from build123d import *

# Parameters (mm, degrees)
SKETCH_R           = 34
SKETCH_R_2         = 27
PAD_DEPTH          = 1.5
SKETCH001_W        = 1.2
SKETCH001_H        = 2
PAD001_DEPTH       = 0.1
SKETCH002_R        = 1
POCKET_DEPTH       = 1.601
SKETCH003_W        = 5
SKETCH003_H        = 5
PAD002_DEPTH       = 1.5
POLARPATTERN_COUNT = 16


with BuildPart() as part:
    # Sketch → Pad (new body)
    with BuildSketch(Plane.XY):
        Circle(SKETCH_R)
        Circle(SKETCH_R_2, mode=Mode.SUBTRACT)
    extrude(amount=PAD_DEPTH)

    # Sketch001 (on Face3 of Pad) → Pad001 (join)
    with BuildSketch(Plane(origin=(0, 0, 0), x_dir=(1, 0, 0), z_dir=(0, 0, -1))):
        with Locations((-3.4, 31.5)):
            Rectangle(SKETCH001_W, SKETCH001_H)
        with Locations((-1.133333, 31.5)):
            Rectangle(SKETCH001_W, SKETCH001_H)
        with Locations((1.133333, 31.5)):
            Rectangle(SKETCH001_W, SKETCH001_H)
        with Locations((3.4, 31.5)):
            Rectangle(SKETCH001_W, SKETCH001_H)
    extrude(amount=PAD001_DEPTH)

    # Sketch002 (on Face3 of Pad001) → Pocket (cut, through all)
    with BuildSketch(Plane.XY.offset(1.5)):
        with Locations((-26.5, 17.5)):
            Circle(SKETCH002_R)
        with Locations((26.5, 17.5)):
            Circle(SKETCH002_R)
        with Locations((26.5, -17.5)):
            Circle(SKETCH002_R)
        with Locations((-26.5, -17.5)):
            Circle(SKETCH002_R)
    extrude(amount=-POCKET_DEPTH, mode=Mode.SUBTRACT)

    # Sketch003 (on Face3 of Pocket) → Pad002 (join)
    with BuildSketch(Plane.XY.offset(1.5)):
        with Locations((0, 29.5)):
            Rectangle(SKETCH003_W, SKETCH003_H)
    pad002 = extrude(amount=PAD002_DEPTH)

    # PolarPattern: Pad002 ×16 about axis
    polarpattern_axis = Axis((0, 0, 1.5), (0, 0, 1))
    for i in range(1, POLARPATTERN_COUNT):
        add(pad002.rotate(polarpattern_axis, i * 360 / POLARPATTERN_COUNT))


solid = part.part
Work out the finished part from the listing and answer in its coordinate system (mm). A direction names the side the tool comes from. Give positions to 0.01 mm unless a question says otherwise; leave off trailing zeros. Loops run counter-clockwise (first coordinate to the right, second up) from the corner with the lowest first, then second, coordinate; pieces in that order, holes last. Notation, with made-up numbers: (31, 9.25) - (72, 9.25) arc R29 ccw to (72, 29.25) - close; hole circle Ø1 at (-23.75, 1.25). An arc over 180 degrees is marked (long way). Answer in a Markdown table with one row per item. Add a question column.
Q1. The part is cut by section B-B (y = 13.5). Determine the outline of the cut face in (x, z).
Q2. Consider line 1 along X through (y, z) = (-29, 2.75); line 2 along X through (y, z) = (1, 0.9); line 3 along Y through (x, z) = (-11, 0.15). Determine where each line is inside the solid, lowest interval first.
Q3. The part is cut by section C-C (x = -23). Determine the outline of the cut face in (y, z).
Q4. A tool of negligible diameter and unlimited length cuts with its end or side. For faces 1 (the flat face through (-22.603, -22.652, 2.24)), 2 (the flat face through (-10.365, 24.931, 2.24)), 3 (the flat face through (22.603, -19.067, 2.24)), 4 (the flat face through (2.5, 29, 2)), 5 (the flat face through (-8.966, -28.179, 2.24)), from which of +Z, -Z, +X, -X, +Y, -Y can it reach the whole face along a straight path? Write none if from no direction.
Q5. Each of these flat-tipped pins is pushed along its axis until it touches: P1, Ø3, axis at x = 26.5, y = 17.5, coming from the +Z side; P2, Ø1.2, axis at x = -26.5, y = 17.5, coming from the -Z side; P3, Ø1.6, axis at x = 30, z = 2, coming from the -Y side; P4, Ø1.6, axis at x = 30.5, z = 2, coming from the +Y side. Where does it stop, or does it pass through?
Q6. Determine the mould class of faces 6 (the flat face through (0, 27, 2)), 7 (the flat face through (30, 0, 3)), 8 (the flat face through (-22.603, 19.067, 2.24)) for opening direction X: released by +X, released by -X, zero draft, split by the parting line, or undercut.
Q7. The part is cut by section A-A (x = -7). Determine the outline of the cut face in (y, z), and give its area (3 significant figures).
Q8. The part is cut by section D-D (y = 5). Determine the outline of the cut face in (x, z).
Solution:
| question | item | result |
|---|---|---|
| 1 | outline | (-31.2, 0) - (-23.38, 0) - (-23.38, 1.5) - (-26.06, 1.5) - (-26.06, 3) - (-29.04, 3) - (-29.04, 1.5) - (-31.2, 1.5) - close; (23.38, 0) - (31.2, 0) - (31.2, 1.5) - (29.04, 1.5) - (29.04, 3) - (26.06, 3) - (26.06, 1.5) - (23.38, 1.5) - close |
| 2 | line 1 | x = -13.61 to -9.31, -2.5 to 2.5, 9.31 to 13.61 |
| 2 | line 2 | x = -33.99 to -26.98, 26.98 to 33.99 |
| 2 | line 3 | y = -32.17 to -24.66, 24.66 to 32.17 |
| 3 | outline | (-25.04, 0) - (-14.14, 0) - (-14.14, 1.5) - (-19.46, 1.5) - (-19.46, 3) - (-22.25, 3) - (-22.25, 1.5) - (-25.04, 1.5) - close; (14.14, 0) - (25.04, 0) - (25.04, 1.5) - (22.25, 1.5) - (22.25, 3) - (19.46, 3) - (19.46, 1.5) - (14.14, 1.5) - close |
| 4 | face 1 | +Z, -X, -Y |
| 4 | face 2 | +Z |
| 4 | face 3 | +Z, +X |
| 4 | face 4 | +Z, +Y, -Y |
| 4 | face 5 | +Z, -Y |
| 5 | P1 | stops at z = 1.5 |
| 5 | P2 | passes through |
| 5 | P3 | stops at y = -17.12 |
| 5 | P4 | stops at y = 16.23 |
| 6 | face 6 | undercut |
| 6 | face 7 | zero draft |
| 6 | face 8 | released by -X |
| 7 | outline | (-33.27, 0) - (-26.08, 0) - (-26.08, 1.5) - (-33.27, 1.5) - close; (26.08, 0) - (33.27, 0) - (33.27, 1.5) - (26.08, 1.5) - close |
| 7 | area | 21.6 mm² |
| 8 | outline | (-33.63, 0) - (-26.53, 0) - (-26.53, 1.5) - (-33.63, 1.5) - close; (26.53, 0) - (33.63, 0) - (33.63, 1.5) - (26.53, 1.5) - close |
